```python
from build123d import *

# Parameters (mm, degrees)
BOSS_EXTRUDE1_DEPTH = 110
BOSS_EXTRUDE2_START = 5.5
SKETCH2_R           = 3
BOSS_EXTRUDE2_DEPTH = 3


with BuildPart() as part:
    # Sketch1 → Boss-Extrude1 (new body)
    with BuildSketch(Plane(origin=(0, 0, 0), x_dir=(1, 0, 0), z_dir=(0, 1, 0))):
        with BuildLine():
            Line((-80, 40.483522574), (-83.3484253, 40.483522574))
            ThreePointArc((-83.3484253, 40.483522574), (0, 92.66), (83.3484253, 40.483522574))
            Line((83.3484253, 40.483522574), (80, 40.483522574))
            ThreePointArc((80, 40.483522574), (0, 89.66), (-80, 40.483522574))
        make_face()
    extrude(amount=BOSS_EXTRUDE1_DEPTH)

    # Sketch2 → Boss-Extrude2 (add)
    # profile 1 of 2: a face of its own
    with BuildSketch(Plane(origin=(0, 0, 0), x_dir=(1, 0, 0), z_dir=(0, 1, 0)).offset(BOSS_EXTRUDE2_START)):
        with BuildLine():
            Line((-80, 40.483522574), (-65, 40.483522574))
            Line((-65, 40.483522574), (-65, 61.756907306))
            ThreePointArc((-65, 61.756907306), (-73.276116331, 51.667459542), (-80, 40.483522574))
        make_face()
        with Locations(Location((-70, 46.483522574, 0), (0, 0, 270))):
            Circle(SKETCH2_R, mode=Mode.SUBTRACT)
    # profile 2 of 2: a face of its own
    with BuildSketch(Plane(origin=(0, 0, 0), x_dir=(1, 0, 0), z_dir=(0, 1, 0)).offset(BOSS_EXTRUDE2_START)):
        with BuildLine():
            Line((80, 40.483522574), (65, 40.483522574))
            Line((65, 40.483522574), (65, 61.756907306))
            ThreePointArc((65, 61.756907306), (73.276116331, 51.667459542), (80, 40.483522574))
        make_face()
        with Locations(Location((70, 46.483522574, 0), (0, 0, 270))):
            Circle(SKETCH2_R, mode=Mode.SUBTRACT)
    extrude(amount=BOSS_EXTRUDE2_DEPTH)


solid = part.part
```
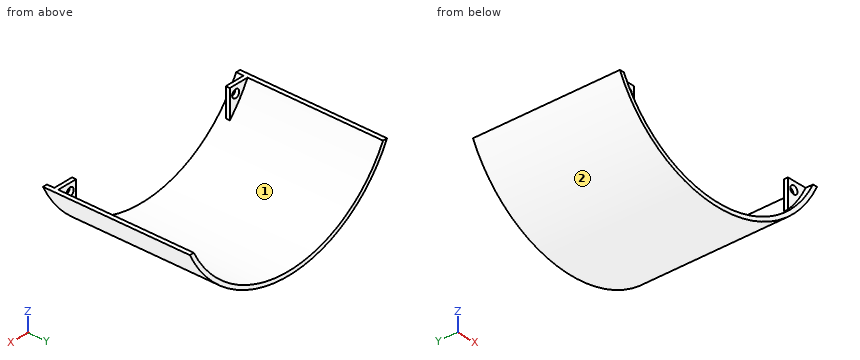
Check sheet for the modelled part. Datum: model origin and axes. Units: mm. Face numbers are marked on the shaded views. Coordinates: 2 decimals unless noted, no trailing zeros. Order: outer loops, then holes, each group sorted by start corner. A loop starts at its lowest first (then second) coordinate and runs counter-clockwise, first axis right, second up. Notation, with made-up numbers: M -6.5,-13.5 L 36.5,-13.5 A32 cw 36.5,15.5 Z; hole C 16.25,-23 d2. An arc over 180 degrees is marked long. Write each question's results on one line, items separated by ' | '. Start each with the question number.
1. Cross-section at A-A on x = -70. Record the cut outline in (y, z), and give its area (3 significant figures).
2. Go/stop test with flat-tipped pins: P1, Ø1, axis at y = 55, z = -81.5, coming from the -X side; P2, Ø12, axis at x = -75, z = -48, coming from the -Y side; P3, Ø6, axis at y = 88.5, z = -53.5, coming from the +X side; P4, Ø1.5, axis at x = 13.5, y = 47, coming from the +Z side. Record where each tip stops, or that it passes through.
3. Cross-section at D-D on y = 25. Record the cut outline in (x, z).
4. Cross-section at C-C on z = -46.5. Record the cut outline in (x, y).
5. Material ranges on probe 1 along X at (y, z) = (7.5, -46.5); probe 2 along X at (y, z) = (6.5, -50.5); probe 3 along X at (y, z) = (16, -64), recorded low to high.
6. Mould release check, pull along X, two halves, no side actions. Record for the marked faces 1 and 2: +X half, -X half, draft (parallel to the pull), parting line (faces both ways), or undercut.
7. Cross-section at B-B on z = -54.5. Record the cut outline in (x, y).
Checks:
1) outline: M 0,-60.71 L 110,-60.71 L 110,-56.03 L 8.5,-56.03 L 8.5,-49.48 L 5.5,-49.48 L 5.5,-56.03 L 0,-56.03 Z; M 5.5,-43.48 L 8.5,-43.48 L 8.5,-40.48 L 5.5,-40.48 Z | area: 544 mm²
2) P1: stops at x = -45 | P2: stops at y = 0 | P3: stops at x = 77.69 | P4: stops at z = -88.52
3) outline: M -83.35,-40.48 A92.66 ccw 83.35,-40.48 L 80,-40.48 A89.66 cw -80,-40.48 Z
4) outline: M -80.15,0 L -76.66,0 L -76.66,5.5 L -73,5.5 L -73,8.5 L -76.66,8.5 L -76.66,110 L -80.15,110 Z; M -67,5.5 L -65,5.5 L -65,8.5 L -67,8.5 Z; M 65,5.5 L 67,5.5 L 67,8.5 L 65,8.5 Z; M 73,5.5 L 76.66,5.5 L 76.66,0 L 80.15,0 L 80.15,110 L 76.66,110 L 76.66,8.5 L 73,8.5 Z
5) probe 1: x = -80.15 to -73, -67 to -65, 65 to 67, 73 to 80.15 | probe 2: x = -77.69 to -65, 65 to 77.69 | probe 3: x = -67.01 to -62.79, 62.79 to 67.01
6) face 1: undercut | face 2: parting line
7) outline: M -74.94,0 L -71.19,0 L -71.19,5.5 L -65,5.5 L -65,8.5 L -71.19,8.5 L -71.19,110 L -74.94,110 Z; M 65,5.5 L 71.19,5.5 L 71.19,0 L 74.94,0 L 74.94,110 L 71.19,110 L 71.19,8.5 L 65,8.5 Z
